Model file for the job. Use its own axes, mm. A direction names the side the tool comes from. Round coordinates to 2 decimals unless told otherwise and drop trailing zeros. Order: outer loops, then holes, each group sorted by start corner. A loop starts at its lowest first (then second) coordinate and runs counter-clockwise, first axis right, second up. Notation, with made-up numbers: (-12, 62.5) - (-6, 62.5) arc R14 ccw to (-6, 74.5) - close; hole circle Ø8 at (-37, 46). An arc over 180 degrees is marked (long way). Write item = value, one per line.
```python
from build123d import *

# Parameters (mm, degrees)
SKETCH1_R           = 3
BOSS_EXTRUDE2_DEPTH = 26.8
SKETCH2_R           = 6.1
CUT_EXTRUDE1_DEPTH  = 26.8
SKETCH3_R           = 6.5
CUT_EXTRUDE2_DEPTH  = 5


with BuildPart() as part:
    # Sketch1 → Boss-Extrude2 (new body)
    with BuildSketch(Plane(origin=(0, 0, 0), x_dir=(1, 0, 0), z_dir=(0, 1, 0))):
        with BuildLine():
            Line((-90, -15), (90, -15))
            ThreePointArc((90, -15), (105, 0), (90, 15))
            Line((90, 15), (-90, 15))
            ThreePointArc((-90, 15), (-105, 0), (-90, -15))
        make_face()
        with Locations(Location((-90, 0, 0), (0, 0, 270))):
            Circle(SKETCH1_R, mode=Mode.SUBTRACT)
        with Locations(Location((90, 0, 0), (0, 0, 270))):
            Circle(SKETCH1_R, mode=Mode.SUBTRACT)
    extrude(amount=BOSS_EXTRUDE2_DEPTH)

    # Sketch2 → Cut-Extrude1 (cut)
    with BuildSketch(Plane.XZ):
        with Locations(Location((90, 0, 0), (0, 0, 270))):
            Circle(SKETCH2_R)
    extrude(amount=-CUT_EXTRUDE1_DEPTH, mode=Mode.SUBTRACT)

    # Sketch3 → Cut-Extrude2 (cut)
    with BuildSketch(Plane.XZ):
        with Locations(Location((90, 0, 0), (0, 0, 270))):
            Circle(SKETCH3_R)
    extrude(amount=-CUT_EXTRUDE2_DEPTH, mode=Mode.SUBTRACT)


solid = part.part
```
1) Mould opens along X. For faces 1 (the face through (96, 5, -2)), 2 (the face through (1, 13, -15)), 3 (the face through (-105, 13, 0)) say: +X half, -X half, draft (parallel to the pull), parting line (faces both ways), or undercut.
Conclusion:
face_1 = undercut
face_2 = draft
face_3 = -X half
2) Flat gauge pins, fed straight in: pin 1 Ø8 at (y, z) = (14, -5.5) entering from -X; pin 2 Ø6 at (y, z) = (12, 9.5) entering from -X. Where does each tip first touch, or does it go through?
Conclusion:
pin_1 = -104.92
pin_2 = -103.52
3) Cut at C-C (z = 12). Write the cut outline in (x, y).
Conclusion:
outline = (-99, 0) - (99, 0) - (99, 26.8) - (-99, 26.8) - close
4) Cut at A-A (z = 0). Write the cut outline in (x, y), and give its area (3 significant figures).
Conclusion:
outline = (-105, 0) - (-93, 0) - (-93, 26.8) - (-105, 26.8) - close; (-87, 0) - (83.5, 0) - (83.5, 5) - (83.9, 5) - (83.9, 26.8) - (-87, 26.8) - close; (96.1, 5) - (96.5, 5) - (96.5, 0) - (105, 0) - (105, 26.8) - (96.1, 26.8) - close
area = 5,140 mm^2
5) Cut at B-B (y = 19). Write the cut outline in (x, z).
Conclusion:
outline = (-90, -15) - (90, -15) arc R15 ccw to (90, 15) - (-90, 15) arc R15 ccw to start; hole circle Ø6 at (-90, 0); hole circle Ø12.2 at (90, 0)
6) 3-axis set-ups, long thin cutter, end or side, ignore diameter. For faces 4 (the face through (83.655, 2.465, 1.409)), 5 (the face through (-1, 0, 0)): which of +Z, -Z, +X, -X, +Y, -Y reach the whole face in a straight line?
Conclusion:
face_4 = -Y
face_5 = +Z, -Z, +X, -X, -Y
7) Wall check: line 1 along X through (y, z) = (14.75, 0); line 2 along X through (y, z) = (2.45, 0); line 3 along X through (y, z) = (2.75, -5). Give the ranges that are in metal, low to high.
Conclusion:
line_1 = -105 to -93, -87 to 83.9, 96.1 to 105
line_2 = -105 to -93, -87 to 83.5, 96.5 to 105
line_3 = -104.14 to 85.85, 94.15 to 104.14
